Could you check a few things on this model? Use its own coordinates, in mm. A direction names the side the tool comes from. Give positions to 0.01 mm unless a question says otherwise; leave off trailing zeros. Write each loop counter-clockwise with the first axis right and the second up, starting at its lowest first coordinate (ties: lowest second). Pieces come first, ordered by that corner, then holes. Notation, with made-up numbers: (-36.75, 26.5) - (11.25, 26.5) arc R5 ccw to (11.25, 31.5) - close; hole circle Ø3 at (11, 53.5). An arc over 180 degrees is marked (long way). Write item = value, one per line.
from build123d import *

# Parameters (mm, degrees)
BASE_DEPTH  = 144
ESQUISSE2_R = 2.5
TROU_DEPTH  = 145.693641878


with BuildPart() as part:
    # Esquisse1 → BASE (new body)
    with BuildSketch(Plane(origin=(0, 0, 0), x_dir=(1, 0, 0), z_dir=(0, 1, 0))):
        Polygon((-2, -3.75), (-2, 2.75), (2, 2.75), (2, -3.75), (12, -3.75), (12, 3.75), (-12, 3.75), (-12, -3.75), align=None)
    extrude(amount=-BASE_DEPTH)

    # Esquisse2 → TROU (cut, through all)
    with BuildSketch(Plane.XY.offset(3.75)):
        with Locations((-7, -8)):
            Circle(ESQUISSE2_R)
        with Locations((7, -8)):
            Circle(ESQUISSE2_R)
        with Locations((7, -24)):
            Circle(ESQUISSE2_R)
        with Locations((7, -40)):
            Circle(ESQUISSE2_R)
        with Locations((7, -56)):
            Circle(ESQUISSE2_R)
        with Locations((7, -72)):
            Circle(ESQUISSE2_R)
        with Locations((7, -88)):
            Circle(ESQUISSE2_R)
        with Locations((7, -104)):
            Circle(ESQUISSE2_R)
        with Locations((7, -120)):
            Circle(ESQUISSE2_R)
        with Locations((7, -136)):
            Circle(ESQUISSE2_R)
        with Locations((-7, -24)):
            Circle(ESQUISSE2_R)
        with Locations((-7, -40)):
            Circle(ESQUISSE2_R)
        with Locations((-7, -56)):
            Circle(ESQUISSE2_R)
        with Locations((-7, -72)):
            Circle(ESQUISSE2_R)
        with Locations((-7, -88)):
            Circle(ESQUISSE2_R)
        with Locations((-7, -104)):
            Circle(ESQUISSE2_R)
        with Locations((-7, -120)):
            Circle(ESQUISSE2_R)
        with Locations((-7, -136)):
            Circle(ESQUISSE2_R)
    extrude(amount=-TROU_DEPTH, mode=Mode.SUBTRACT)


solid = part.part
1. Thinking about a two-plate mould opening in Y: for faces 3 (the face through (6.67, -85.52, 0.05)), 4 (the face through (2.5, 0, -0.1)), 5 (the face through (12, -71, 0)), which applies, pulls with the +Y half, pulls with the -Y half, needs draft (parallel to the pull), parting line crosses it, or undercut?
Filled sheet:
face_3 = undercut
face_4 = pulls with the +Y half
face_5 = needs draft
2. If we section it at C-C, the plane y = -60: Please give me the cut outline in (x, z).
Filled sheet:
outline = (-12, -3.75) - (12, -3.75) - (12, 3.75) - (2, 3.75) - (2, -2.75) - (-2, -2.75) - (-2, 3.75) - (-12, 3.75) - close
3. I need wall thicknesses on line 1 (X direction, y = -74, z = -2); line 2 (X direction, y = -14.5, z = 2.75); line 3 (X direction, y = -73, z = 0). Which ranges of each line are inside material? Lowest first, please.
Filled sheet:
line_1 = -12 to -8.5, -5.5 to -2, 2 to 5.5, 8.5 to 12
line_2 = -12 to -2, 2 to 12
line_3 = -12 to -9.29, -4.71 to -2, 2 to 4.71, 9.29 to 12
4. If we section it at A-A, the plane z = 2: Count the separate pieces of the cut face and the enclosed holes in it, and give its area (3 significant figures).
Filled sheet:
separate_pieces = 2
enclosed_holes = 18
area = 2,530 mm2
5. Which directions (+Z, -Z, +X, -X, +Y, -Y) give clear straight access to the entire face, cutting with the end or side of a thin tool? Please do faces 1 (the face through (-2, -71, 1)), 2 (the face through (-7.33, -85.52, 0.05)).
Filled sheet:
face_1 = +Z, +Y, -Y
face_2 = +Z, -Z
6. If we section it at B-B, the plane y = -88: Please give me the cut outline in (x, z), and give its area (3 significant figures).
Filled sheet:
outline = (-12, -3.75) - (-9.5, -3.75) - (-9.5, 3.75) - (-12, 3.75) - close; (-4.5, -3.75) - (4.5, -3.75) - (4.5, 3.75) - (2, 3.75) - (2, -2.75) - (-2, -2.75) - (-2, 3.75) - (-4.5, 3.75) - close; (9.5, -3.75) - (12, -3.75) - (12, 3.75) - (9.5, 3.75) - close
area = 79.0 mm2
